```python
from build123d import *

# Parameters (mm, degrees)
F_1_8_0_125_DIAMETER_HOLE1_D     = 3.175
F_1_8_0_125_DIAMETER_HOLE1_DEPTH = 15.875
F_1_8_0_125_DIAMETER_HOLE1_TIP   = 0.953866233


with BuildPart() as part:
    # Sketch1 → Revolve1 (revolve)
    with BuildSketch(Plane(origin=(0, 0, 0), x_dir=(0, 0, -1), z_dir=(1, 0, 0))):
        Polygon((0, 0), (-9.398, 0), (-9.398, 19.05), (-12.7, 19.05), (-12.7, 22.225), (12.7, 22.225), (12.7, 19.05), (9.398, 19.05), (9.398, 0), align=None)
    revolve(axis=Axis((0, 0, 0), (0, 0, 1)))

    # 1/8 (0.125) Diameter Hole1
    with Locations(Plane(origin=(0, -22.225, 0), x_dir=(-1, 0, 0), z_dir=(0, -1, 0))):
        with Locations((0, 0)):
            Hole(F_1_8_0_125_DIAMETER_HOLE1_D / 2, depth=F_1_8_0_125_DIAMETER_HOLE1_DEPTH)
            with Locations((0, 0, -(F_1_8_0_125_DIAMETER_HOLE1_DEPTH + F_1_8_0_125_DIAMETER_HOLE1_TIP / 2))):  # 118° drill point
                Cone(0, F_1_8_0_125_DIAMETER_HOLE1_D / 2, F_1_8_0_125_DIAMETER_HOLE1_TIP, mode=Mode.SUBTRACT)


solid = part.part
```
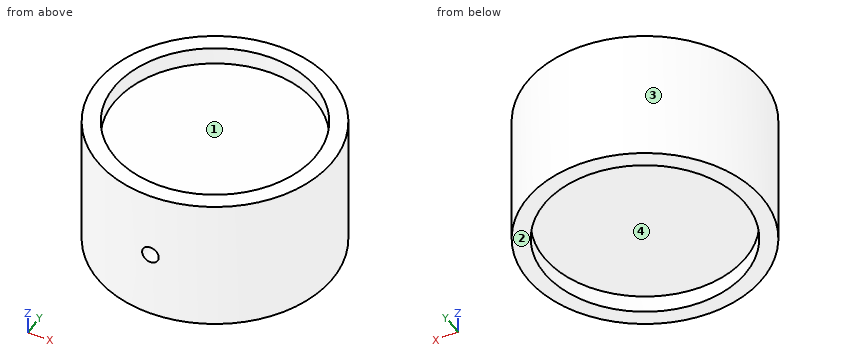
Build history of the part. All positions in model axes, mm. Face numbers are marked on the shaded views. Give positions to 0.01 mm unless a question says otherwise; leave off trailing zeros. Loops run counter-clockwise (first coordinate to the right, second up) from the corner with the lowest first, then second, coordinate; pieces in that order, holes last.
1) Two-plate mould, pull along X, no slides. Class the marked faces 1, 2, 3 and 4: released by +X, released by -X, zero draft, split by the parting line, or undercut.
Values follow:
face 1: undercut
face 2: zero draft
face 3: split by the parting line
face 4: undercut
2) Probe line 1 along X through (y, z) = (0, -10.05) (3 decimals); line 2 along Z through (x, y) = (0, -18); line 3 along Z through (x, y) = (4, 7). List the from-to ranges inside material, lowest first.
Values follow:
line 1: x = -22.225 to -19.05, 19.05 to 22.225
line 2: z = -9.4 to -1.59, 1.59 to 9.4
line 3: z = -9.4 to 9.4
3) Band-saw the part on C-C on y = -8.5. List the corners of the cut face in (x, z) (1 decimal), then the cut area to 3 significant figures.
Values follow:
outline: (-20.5, -12.7) - (-17, -12.7) - (-17, -9.4) - (17, -9.4) - (17, -12.7) - (20.5, -12.7) - (20.5, 12.7) - (17, 12.7) - (17, 9.4) - (-17, 9.4) - (-17, 12.7) - (-20.5, 12.7) - close; hole circle Ø3.2 at (0, 0)
area: 810 mm2
4) Band-saw the part on B-B on x = -12.5. List the corners of the cut face in (y, z), then the cut area to 3 significant figures.
Values follow:
outline: (-18.38, -12.7) - (-14.38, -12.7) - (-14.38, -9.4) - (14.38, -9.4) - (14.38, -12.7) - (18.38, -12.7) - (18.38, 12.7) - (14.38, 12.7) - (14.38, 9.4) - (-14.38, 9.4) - (-14.38, 12.7) - (-18.38, 12.7) - close
area: 744 mm2
5) Band-saw the part on D-D on z = -2.75. List the corners of the cut face in (x, y) (3 decimals), then the cut area to 3 significant figures.
Values follow:
outline: circle Ø44.45 at (0, 0)
area: 1,550 mm2
6) Drop flat-ended pins along their axis: P1, Ø8, axis at y = 3.5, z = 3, coming from the +X side (3 decimals); P2, Ø8, axis at y = -17.5, z = -8, coming from the -X side; P3, Ø12, axis at x = 12.5, z = 3.5, coming from the +Y side; P4, Ø12, axis at x = -17, y = -7.5, coming from the +Z side. Give the stop position or say it passes through.
Values follow:
P1: stops at x = 22.225
P2: stops at x = -17.66
P3: stops at y = 21.25
P4: stops at z = 12.7
7) Band-saw the part on A-A on y = 0. List the corners of the cut face in (x, z) (3 decimals).
Values follow:
outline: (-22.225, -12.7) - (-19.05, -12.7) - (-19.05, -9.398) - (19.05, -9.398) - (19.05, -12.7) - (22.225, -12.7) - (22.225, 12.7) - (19.05, 12.7) - (19.05, 9.398) - (-19.05, 9.398) - (-19.05, 12.7) - (-22.225, 12.7) - close
